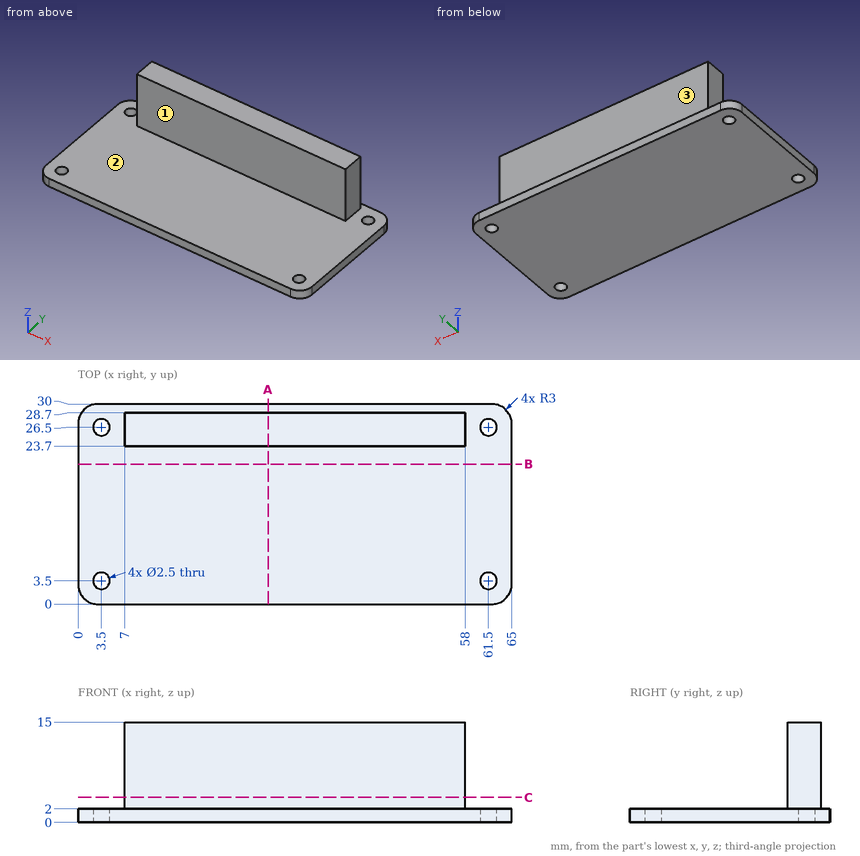
Here's the drawing with two shaded views (mm, measured from the low corner). I have some questions. Give positions to 0.01 mm unless a question says otherwise; leave off trailing zeros. Write each loop counter-clockwise with the first axis right and the second up, starting at its lowest first coordinate (ties: lowest second). Pieces come first, ordered by that corner, then holes. Notation, with made-up numbers: (45.25, 50) - (55.25, 50) arc R16 cw to (55.25, 55) - close; hole circle Ø10 at (65, 21). An arc over 180 degrees is marked (long way). One line per item, written item: value. Start each with the question number.
Item 1: Imagine slicing it at A-A, the plane x = 28.5. List the corners of the cut face in (y, z) for me, and give its area (3 significant figures).
Item 2: Imagine slicing it at C-C, the plane z = 3.75. List the corners of the cut face in (x, y) for me, and give its area (3 significant figures).
Item 3: I'm going to push flat-ended pins straight in: pin 1 (8 mm diameter, centred on x = 14.5, y = 18.5, fed in from +Z); pin 2 (4 mm diameter, centred on y = 20, z = 11, fed in from -X); pin 3 (2.5 mm diameter, centred on y = 27.5, z = 8, fed in from -X); pin 4 (4 mm diameter, centred on x = 32, z = 7, fed in from -Y). Where does each tip first touch, or does it pass through?
Item 4: Please list where these lines run through material, in increasing order: line 1 (Y direction, x = 61.5, z = 1.3); line 2 (Z direction, x = 5, y = 13.5); line 3 (Y direction, x = 41.5, z = 10.5). Write a range as from..to.
Item 5: If we mould it in two halves opening along Y, with no side actions, what happens to the marked faces 1, 2 and 3? For each: +Y half, -Y half, draft (parallel to the pull), parting line (faces both ways), or undercut.
Item 6: Imagine slicing it at B-B, the plane y = 21. List the corners of the cut face in (x, z) for me.
Geometry says:
1. outline: (0, 0) - (30, 0) - (30, 2) - (28.7, 2) - (28.7, 15) - (23.7, 15) - (23.7, 2) - (0, 2) - close
1. area: 125 mm^2
2. outline: (7, 23.7) - (58, 23.7) - (58, 28.7) - (7, 28.7) - close
2. area: 255 mm^2
3. pin 1: z = 2
3. pin 2: through
3. pin 3: x = 7
3. pin 4: y = 23.7
4. line 1: 0..2.25, 4.75..25.25, 27.75..30
4. line 2: 0..2
4. line 3: 23.7..28.7
5. face 1: -Y half
5. face 2: draft
5. face 3: +Y half
6. outline: (0, 0) - (65, 0) - (65, 2) - (0, 2) - close
